Geometry: final body of the model. Coordinates: model frame, mm. Face numbers are marked on the shaded views. A direction names the side the tool comes from. Coordinates: 2 decimals unless noted, no trailing zeros. Write each loop counter-clockwise with the first axis right and the second up, starting at its lowest first coordinate (ties: lowest second). Pieces come first, ordered by that corner, then holes. Notation, with made-up numbers: (-19.75, 89) - (-9.75, 89) arc R15 ccw to (-9.75, 102) - close; hole circle Ø3 at (60, 7.5). An arc over 180 degrees is marked (long way). Put each result on its own line as item: value.
Autodesk Inventor part; units mm, degrees
ref_plane "РабПлоскость1" through (27.2, 11.2, 3) normal (1, 0, 0) x (0, 0, -1)
ref_plane "YZ Plane" through (0, 0, 0) normal (1, 0, 0) x (0, 1, 0)
ref_plane "XZ Plane" through (0, 0, 0) normal (0, 1, 0) x (-1, 0, 0)
sketch "Эскиз1" plane through (0, 0, 0) normal (0, 0, 1) x (1, 0, 0)
  line L0 (0, 0) -> (5, 0)
  line L1 (5, 0) -> (5, 7)
  line L2 (5, 7) -> (0, 7)
  line L3 (0, 7) -> (0, 0)
  line L4 (0, 0) -> (27.2, 0)
  line L5 (27.2, 0) -> (27.2, -5)
  line L6 (27.2, -5) -> (0, -5)
  line L7 (0, -5) -> (0, 0)
  dimension "d0" = 5
  dimension "d1" = 7
  dimension "d2" = 27.2
  dimension "d3" = 5
extrude "Выдавливание1" add sketch "Эскиз1" along normal blind 6
sketch "Эскиз4" plane through (0, 7, 0) normal (0, 1, 0) x (1, 0, 0)
  line L0 (0, 0) -> (0, -6)
  line L1 (0, 0) -> (0, -6)
  line L2 (5, 0) -> (0, 0)
  line L3 (0, 0) -> (0, -6)
  line L4 (5, -6) -> (0, -6)
  line L5 (5, 0) -> (5, -6)
  point P0 (0, -6)
  point P1 (0, 0)
extrude "Выдавливание2" add sketch "Эскиз4" along normal blind 7.2
fillet "Сопряжение1" radius 3 2 edges at (2.5, 14.2, 6) (2.5, 14.2, 0)
sketch "Эскиз5" plane through (5, 0, 6) normal (1, 0, 0) x (0, 0, -1)
  line L0 (0, -5) -> (0, -5)
  arc A0 (6, 11.2) -> (0, 11.2) centre (3, 11.2) ccw
  point P0 (6, 0)
  point P1 (6, -5)
  point P2 (2.5, 25.2)
hole "Отверстие2" at (5, 11.2, 3) direction (-1, 0, 0) diameter 3.2 depth 5
mirror "Зеркальное отражение1" about plane through (27.2, -5, 0) normal (1, 0, 0)
sketch "Эскиз9" plane through (0, 0, 0) normal (0, 0, -1) x (-1, 0, 0)
  line L0 (0, -5) -> (-54.4, -5)
  line L1 (-54.4, 11.2) -> (-54.4, -5)
  line L2 (-54.4, -5) -> (-43.75, -61.25)
  line L3 (-43.75, -61.25) -> (-43.75, -69.75)
  line L4 (-43.75, -69.75) -> (-36.75, -69.75)
  line L5 (-36.75, -69.75) -> (-36.75, -61.25)
  line L6 (-36.75, -61.25) -> (-47.4, -5)
  point P0 (0, 0)
  dimension "d82" = 64.75
  dimension "d83" = 7
  dimension "d86" = 8.5
  dimension "d95" = 10.65
extrude "Выдавливание4" add sketch "Эскиз9" against normal blind 6
sketch "Эскиз11" plane through (0, 0, 6) normal (0, 0, 1) x (1, 0, 0)
  line L0 (40.25, -69.75) -> (40.25, -64.8)
  line L1 (36.75, -69.75) -> (43.75, -69.75)
  point P0 (0, 0)
  dimension "d91" = 4.95
hole "Отверстие6" at (40.25, -64.8, 6) direction (0, 0, -1) diameter 3.2 end through all
ref_plane "РабПлоскость1" through (27.2, 11.2, 3) normal (1, 0, 0) x (0, 0, -1)
mirror "Зеркальное отражение2" about plane through (27.2, 11.2, 3) normal (1, 0, 0) of "Выдавливание4", "Отверстие6"
fillet "Сопряжение3" radius 6 8 edges at (43.75, -61.25, 3) (36.75, -61.25, 3) (17.65, -61.25, 3) (10.65, -61.25, 3) (0, -5, 3) (7, -5, 3) (47.4, -5, 3) (54.4, -5, 3)
equation "\"Радиус_гибки\" = Толщина"
equation "\"Ширина_просечки\" = Толщина"
equation "\"Глубина_просечки\" = 0.5 * Толщина"
equation "\"Размер_просечки\" = 4 * Толщина"
equation "\"Мин_остаток\" = 2 * Толщина"
equation "\"Радиус_перехода\" = Радиус_гибки"
equation "\"Радиус_Якоби\" = Толщина"
equation "\"Размер_зазора\" = Толщина"
properties part number "Стойка для камеры"
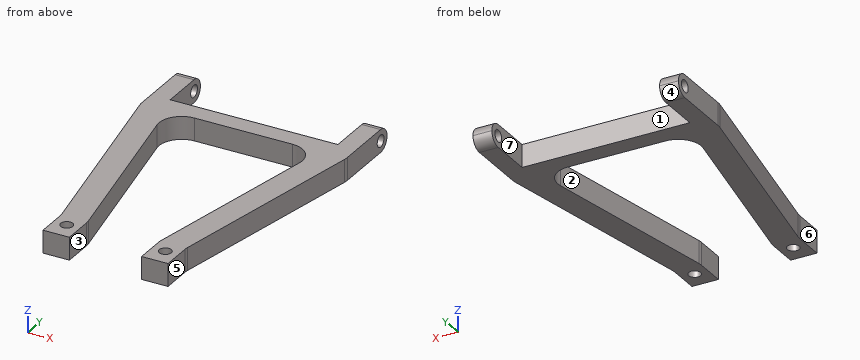
1. Pin query (flat end, axial travel): pin 1 Ø3 at (y, z) = (-65.5, 4.5) entering from +X; pin 2 Ø2.5 at (x, y) = (40.25, -64.8) entering from -Z; pin 3 Ø3 at (x, z) = (31, 4.5) entering from +Y; pin 4 Ø1.5 at (y, z) = (-23, 3.5) entering from -X. Return the tip coordinate at first contact, or that it passes through.
Answer below:
pin 1: stops at x = 43.75
pin 2: passes through
pin 3: stops at y = 0
pin 4: stops at x = 3.27
2. Section query C-C (y = -43.5). Return loops of the section in (x, z), then the cut area to 3 significant figures.
Answer below:
outline: (7.29, 0) - (14.29, 0) - (14.29, 6) - (7.29, 6) - close; (40.11, 0) - (47.11, 0) - (47.11, 6) - (40.11, 6) - close
area: 84.0 mm²
3. Section query A-A (y = -64.8). Return loops of the section in (x, z).
Answer below:
outline: (10.65, 0) - (12.55, 0) - (12.55, 6) - (10.65, 6) - close; (15.75, 0) - (17.65, 0) - (17.65, 6) - (15.75, 6) - close; (36.75, 0) - (38.65, 0) - (38.65, 6) - (36.75, 6) - close; (41.85, 0) - (43.75, 0) - (43.75, 6) - (41.85, 6) - close
4. Section query B-B (x = 30). Return loops of the section in (y, z).
Answer below:
outline: (-5, 0) - (0, 0) - (0, 6) - (-5, 6) - close
5. Mould query, pull axis X, two halves, no side actions, for the marked faces 4, 5, 6 and 7. Classes: +X half, -X half, draft (parallel to the pull), parting line (faces both ways), or undercut.
Answer below:
face 4: draft
face 5: +X half
face 6: -X half
face 7: undercut
6. Section query D-D (x = 47). Return loops of the section in (y, z).
Answer below:
outline: (-44.08, 0) - (0, 0) - (0, 6) - (-44.08, 6) - close
7. Ray query, probe 1 along X at (y, z) = (-64.8, 2.1); probe 2 along Z at (x, y) = (2, 11); probe 3 along X at (y, z) = (2.5, 1.7). Return the intervals inside material, ascending. Write a range as from..to.
Answer below:
probe 1: x = 10.65..12.55, 15.75..17.65, 36.75..38.65, 41.85..43.75
probe 2: z = 0..1.41, 4.59..6
probe 3: x = 0..5, 49.4..54.4
8. Set-up query: the marked faces 1, 2 and 3. Return all of +Z, -Z, +X, -X, +Y, -Y with unobstructed straight access to the full face (end or side cutting, diameter ignored); none if empty.
Answer below:
face 1: +Z, -Z, +Y
face 2: +Z, -Z
face 3: +Z, -Z, -Y
